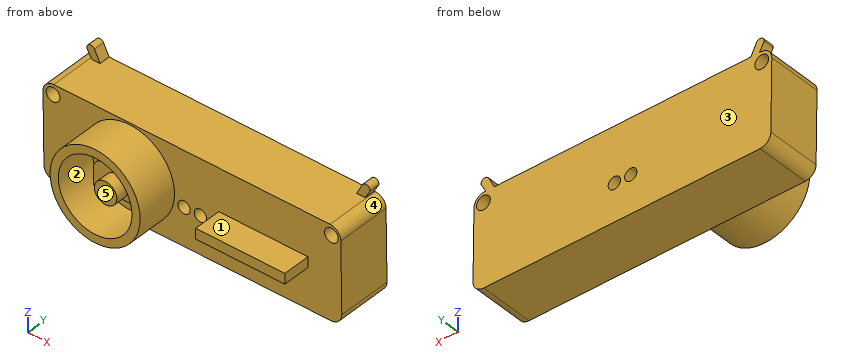
```python
from build123d import *

# Parameters (mm, degrees)
F0_R      = 2.895724
F0_R_2    = 3.241562
F1_DEPTH  = 25.4
F2_R      = 5.08
F3_DEPTH  = 5.08
F5_DEPTH  = 32.3342
F6_R      = 5.08
F7_R      = 5.276508
F8_DEPTH  = 38.354
F9_R      = 21.156257
F9_R_2    = 17.306623
F10_DEPTH = 44.704
F12_DEPTH = 38.354


with BuildPart() as f1:
    # F0 (on Front) → F1 (new body)
    with BuildSketch(Plane.XZ):
        Polygon((70.342824, -21.445718), (69.763908, 21.972595), (64.276244, 21.972595), (60.254056, 21.972595), (-60.254056, 21.972595), (-64.276244, 21.972595), (-70.167677, 21.972595), (-69.607526, -21.638222), align=None)
        with Locations((-3.860941, -3.798458)):
            Circle(F0_R, mode=Mode.SUBTRACT)
        with Locations((3.860941, -3.798458)):
            Circle(F0_R, mode=Mode.SUBTRACT)
        with Locations((-65.373771, 17.245404)):
            Circle(F0_R_2, mode=Mode.SUBTRACT)
        with Locations((65.373771, 17.245404)):
            Circle(F0_R_2, mode=Mode.SUBTRACT)
    extrude(amount=F1_DEPTH)

    # F2
    f2_edges = [f1.edges().sort_by_distance(p)[0] for p in [
        (69.763908, -12.7, 21.972595),
        (-70.167677, -12.7, 21.972595),
        (-69.607526, -12.7, -21.638222),
        (70.342824, -12.7, -21.445718),
    ]]
    fillet(f2_edges, radius=F2_R)

    # F0 (on Front) → F3 (join)
    with BuildSketch(Plane.XZ):
        with BuildLine():
            Line((-64.276244, 21.972595), (-60.254056, 21.972595))
            Line((-60.254056, 21.972595), (-62.904059, 27.139447))
            ThreePointArc((-62.904059, 27.139447), (-65.222607, 28.088801), (-66.516974, 25.943679))
            Line((-66.516974, 25.943679), (-64.276244, 21.972595))
        make_face()
        with BuildLine():
            Line((60.254056, 21.972595), (64.276244, 21.972595))
            Line((64.276244, 21.972595), (66.516974, 25.943679))
            ThreePointArc((66.516974, 25.943679), (65.222607, 28.088801), (62.904059, 27.139447))
            Line((62.904059, 27.139447), (60.254056, 21.972595))
        make_face()
    extrude(amount=F3_DEPTH)

    # F4 (on Front) → F5 (join)
    with BuildSketch(Plane.XZ):
        Polygon((-19.896746, 5.259533), (-40.63455, 5.259533), (-40.63455, -7.440129), (-19.802189, -7.440129), align=None)
    extrude(amount=F5_DEPTH)

    # F6
    f6_edges = [f1.edges().sort_by_distance(p)[0] for p in [
        (-40.63455, -28.8671, 5.259533),
        (-19.896746, -28.8671, 5.259533),
    ]]
    fillet(f6_edges, radius=F6_R)

    # F7 (on Front) → F8 (join)
    with BuildSketch(Plane.XZ):
        with Locations((-29.851345, -2.50347)):
            Circle(F7_R)
    extrude(amount=F8_DEPTH)

    # F9 (on Front) → F10 (join)
    with BuildSketch(Plane.XZ):
        with Locations((-29.464282, 0)):
            Circle(F9_R)
        with Locations((-29.464282, 0)):
            Circle(F9_R_2, mode=Mode.SUBTRACT)
    extrude(amount=F10_DEPTH)

    # F11 (on Front) → F12 (join)
    with BuildSketch(Plane.XZ):
        Polygon((54.370172, 2.222606), (12.467819, 2.222606), (12.476523, -2.632661), (54.370172, -2.632661), align=None)
    extrude(amount=F12_DEPTH)


solid = f1.part
```
Model file for the job. Use its own axes, mm. Face numbers are marked on the shaded views. A direction names the side the tool comes from. Round coordinates to 2 decimals unless told otherwise and drop trailing zeros. Order: outer loops, then holes, each group sorted by start corner. A loop starts at its lowest first (then second) coordinate and runs counter-clockwise, first axis right, second up. Notation, with made-up numbers: M 40,46 L 54,46 A17 ccw 54,75 Z; hole C 62,66.5 d2. An arc over 180 degrees is marked long. Use CSV: the item, a comma, the result in double quotes.
Item 1: Pin check, flat tips, straight feed: pin 1 (6 mm diameter, centred on x = 28.5, z = -16, fed in from -Y); pin 2 (7.5 mm diameter, centred on x = 65.37, z = 17.25, fed in from +Y); pin 3 (4 mm diameter, centred on x = 42, y = -38.5, fed in from -Z); pin 4 (5.5 mm diameter, centred on x = -36.5, y = -28, fed in from -Z). Stop position of each tip, or through.
Worked answers:
pin 1,"y = -25.4"
pin 2,"y = 0"
pin 3,"z = -2.63"
pin 4,"z = -21.59"
Item 2: Saw through at A-A (y = -30). List the corners of the cut face in (x, z), plus the area to 3 significant figures.
Worked answers:
outline,"C -29.46,0 d42.31; M -40.63,-7.44 L -31.71,-7.44 A5.28 ccw -27.99,-7.44 L -19.8,-7.44 L -19.86,0.22 A5.08 ccw -24.94,5.26 L -35.55,5.26 A5.08 ccw -40.63,0.18 Z; M 12.47,2.22 L 12.48,-2.63 L 54.37,-2.63 L 54.37,2.22 Z; hole C -29.46,0 d34.61"
area,"922 mm²"
Item 3: Pull direction X, two halves, no side cores. Call the marked faces 3, 4 and 5: released by +X, released by -X, zero draft, split by the parting line, or undercut.
Worked answers:
face 3,"zero draft"
face 4,"released by +X"
face 5,"undercut"
Item 4: Saw through at B-B (y = -20). List the corners of the cut face in (x, z), plus the area to 3 significant figures.
Worked answers:
outline,"M -70.1,16.83 L -69.67,-16.62 A5.08 ccw -64.59,-21.63 L 65.2,-21.45 A5.08 ccw 70.27,-16.31 L 69.83,16.96 A5.08 ccw 64.75,21.97 L -65.02,21.97 A5.08 ccw Z; hole C -65.37,17.25 d6.48; hole C -3.86,-3.8 d5.79; hole C 3.86,-3.8 d5.79; hole C 65.37,17.25 d6.48"
area,"5,950 mm²"
Item 5: Saw through at C-C (z = -11.5). List the corners of the cut face in (x, y), plus the area to 3 significant figures.
Worked answers:
outline,"M -69.74,-25.4 L -47.22,-25.4 L -47.22,-44.7 L -42.4,-44.7 L -42.4,-25.4 L -16.53,-25.4 L -16.53,-44.7 L -11.71,-44.7 L -11.71,-25.4 L 70.21,-25.4 L 70.21,0 L -69.74,0 Z"
area,"3,740 mm²"
Item 6: Which spindle directions (+Z, -Z, +X, -X, +Y, -Y) get a long thin tool onto all of the face, cutting with end or side? Do the marked faces 1 and 2. Say none if no direction does.
Worked answers:
face 1,"+Z, +X, -Y"
face 2,"-Y"
Item 7: Probe probe 1 along X at (y, z) = (-40.5, 0); probe 2 along X at (y, z) = (-4.5, -2.5); probe 3 along Y at (x, z) = (-54, 4). List the from-to ranges inside material, lowest first.
Worked answers:
probe 1,"-50.62 to -46.77, -12.16 to -8.31"
probe 2,"-69.85 to -6.45, -1.27 to 1.27, 6.45 to 70.09"
probe 3,"-25.4 to 0"
Item 8: Saw through at D-D (y = -40). List the corners of the cut face in (x, z), plus the area to 3 significant figures.
Worked answers:
outline,"C -29.46,0 d42.31; hole C -29.46,0 d34.61"
area,"465 mm²"
